Input: part model. Units: mm. Frame: model coordinates. A direction names the side the tool comes from. Give positions to 0.01 mm unless a question says otherwise; leave off trailing zeros. Loops run counter-clockwise (first coordinate to the right, second up) from the corner with the lowest first, then second, coordinate; pieces in that order, holes last. Notation, with made-up numbers: (87.25, 7) - (104.25, 7) arc R22 ccw to (104.25, 45) - close; hole circle Ø6 at (45.5, -37.5). An arc over 180 degrees is marked (long way). Answer as a JSON object with one key per item and string values.
from build123d import *

# Parameters (mm, degrees)
SKETCH1_7_W         = 63
SKETCH1_7_H         = 55
SKETCH1_7_R         = 1.5
SKETCH1_7_R_2       = 11.375
BOSS_EXTRUDE3_DEPTH = 10
BOSS_EXTRUDE4_START = -65
SKETCH1_8_W         = 63
SKETCH1_8_H         = 55
SKETCH1_8_R         = 1.5
SKETCH1_8_W_2       = 43
SKETCH1_8_H_2       = 43
BOSS_EXTRUDE4_DEPTH = 65
SKETCH4_W           = 12.5
SKETCH4_H           = 65
CUT_EXTRUDE5_DEPTH  = 6
SKETCH1_15_R        = 11.375
SKETCH1_15_R_2      = 4.375
BOSS_EXTRUDE5_DEPTH = 7
SKETCH1_16_R        = 11.375
SKETCH1_16_R_2      = 4.375
CUT_EXTRUDE7_DEPTH  = 3


with BuildPart() as part:
    # Sketch1<7> → Boss-Extrude3 (new body)
    with BuildSketch(Plane.XY):
        with Locations((21.5, 21.5)):
            Rectangle(SKETCH1_7_W, SKETCH1_7_H)
        with Locations((-5, 36.5)):
            Circle(SKETCH1_7_R, mode=Mode.SUBTRACT)
        with Locations((-5, 6.5)):
            Circle(SKETCH1_7_R, mode=Mode.SUBTRACT)
        with Locations((48, 6.5)):
            Circle(SKETCH1_7_R, mode=Mode.SUBTRACT)
        with Locations((48, 36.5)):
            Circle(SKETCH1_7_R, mode=Mode.SUBTRACT)
        with Locations((21.5, 21.5)):
            Circle(SKETCH1_7_R_2, mode=Mode.SUBTRACT)
    extrude(amount=BOSS_EXTRUDE3_DEPTH)

    # Sketch1<8> → Boss-Extrude4 (add)
    with BuildSketch(Plane.XY.offset(BOSS_EXTRUDE4_START)):
        with Locations((21.5, 21.5)):
            Rectangle(SKETCH1_8_W, SKETCH1_8_H)
        with Locations((48, 6.5)):
            Circle(SKETCH1_8_R, mode=Mode.SUBTRACT)
        with Locations((-5, 6.5)):
            Circle(SKETCH1_8_R, mode=Mode.SUBTRACT)
        with Locations((-5, 36.5)):
            Circle(SKETCH1_8_R, mode=Mode.SUBTRACT)
        with Locations((48, 36.5)):
            Circle(SKETCH1_8_R, mode=Mode.SUBTRACT)
        with Locations((21.5, 21.5)):
            Rectangle(SKETCH1_8_W_2, SKETCH1_8_H_2, mode=Mode.SUBTRACT)
    extrude(amount=BOSS_EXTRUDE4_DEPTH)

    # Sketch4 → Cut-Extrude5 (cut)
    with BuildSketch(Plane.XZ.offset(-43)):
        with Locations((27.75, -32.5)):
            Rectangle(SKETCH4_W, SKETCH4_H)
        with Locations((15.25, -32.5)):
            Rectangle(SKETCH4_W, SKETCH4_H)
    extrude(amount=-CUT_EXTRUDE5_DEPTH, mode=Mode.SUBTRACT)

    # Sketch1<15> → Boss-Extrude5 (add)
    with BuildSketch(Plane.XY):
        with Locations((21.5, 21.5)):
            Circle(SKETCH1_15_R)
        with Locations((21.5, 21.5)):
            Circle(SKETCH1_15_R_2, mode=Mode.SUBTRACT)
    extrude(amount=BOSS_EXTRUDE5_DEPTH)

    # Sketch1<16> → Cut-Extrude7 (cut)
    with BuildSketch(Plane.XY):
        with Locations((21.5, 21.5)):
            Circle(SKETCH1_16_R)
        with Locations((21.5, 21.5)):
            Circle(SKETCH1_16_R_2, mode=Mode.SUBTRACT)
    extrude(amount=CUT_EXTRUDE7_DEPTH, mode=Mode.SUBTRACT)


solid = part.part
Item 1: Cut plane D-D (y = 36.5). Return loops of the section in (x, z).
Geometry check:
{"outline": "(-10, -65) - (-6.5, -65) - (-6.5, 10) - (-10, 10) - close; (-3.5, -65) - (0, -65) - (0, 0) - (43, 0) - (43, -65) - (46.5, -65) - (46.5, 10) - (-3.5, 10) - close; (49.5, -65) - (53, -65) - (53, 10) - (49.5, 10) - close"}
Item 2: Material intervals for line 1 (Y direction, x = -5, z = -30); line 2 (X direction, y = 23.5, z = -30); line 3 (Y direction, x = 21.5, z = 1.8) (3 decimals), sorted ascending. Write a range as [from, to].
Geometry check:
{"line 1": "y = [-6, 5], [8, 35], [38, 49]", "line 2": "x = [-10, 0], [43, 53]", "line 3": "y = [-6, 10.125], [32.875, 49]"}
Item 3: Cut plane A-A (x = -5). Return loops of the section in (y, z).
Geometry check:
{"outline": "(-6, -65) - (5, -65) - (5, 10) - (-6, 10) - close; (8, -65) - (35, -65) - (35, 10) - (8, 10) - close; (38, -65) - (49, -65) - (49, 10) - (38, 10) - close"}
Item 4: Access query for faces 5 (the face through (9, 46, -33)), 6 (the face through (13.12, 29.19, 1.48)), 7 (the face through (-10, 21, -28)), 8 (the face through (26, 22, 7)). Directions: +Z, -Z, +X, -X, +Y, -Y. A direction counts if a zero-diameter tool reaches every point of the face in a straight line with its end or side. Return the directions, or none.
Geometry check:
{"face 5": "-Z, +Y", "face 6": "-Z", "face 7": "+Z, -Z, -X, +Y, -Y", "face 8": "+Z"}
Item 5: Mould query, pull axis Y, two halves, no side actions, for faces 1 (the face through (21, 34, 10)), 2 (the face through (26, 22, 3)), 3 (the face through (-5, 35, -28)), 4 (the face through (7, 49, -28)). Classes: released by +Y, released by -Y, zero draft, split by the parting line, or undercut.
Geometry check:
{"face 1": "zero draft", "face 2": "undercut", "face 3": "undercut", "face 4": "released by +Y"}
Item 6: Cut plane B-B (y = 21.5). Return loops of the section in (x, z) (3 decimals).
Geometry check:
{"outline": "(-10, -65) - (0, -65) - (0, 0) - (10.125, 0) - (10.125, 3) - (17.125, 3) - (17.125, 7) - (10.125, 7) - (10.125, 10) - (-10, 10) - close; (25.875, 3) - (32.875, 3) - (32.875, 0) - (43, 0) - (43, -65) - (53, -65) - (53, 10) - (32.875, 10) - (32.875, 7) - (25.875, 7) - close"}
Item 7: Contact query for flat-ended pins moving along their axis: P1, Ø11.5, axis at x = 26, y = 17, coming from the -Z side; P2, Ø13.5, axis at x = 21.5, y = 21.5, coming from the -Z side; P3, Ø4, axis at x = 27, z = -30, coming from the +Y side. Output: stop coordinate, or through.
Geometry check:
{"P1": "stops at z = 0", "P2": "stops at z = 3", "P3": "stops at y = 0"}
Item 8: Cut plane C-C (x = 21.5). Return loops of the section in (y, z) (3 decimals), then the cut area to 4 significant figures.
Geometry check:
{"outline": "(-6, -65) - (0, -65) - (0, 0) - (10.125, 0) - (10.125, 3) - (17.125, 3) - (17.125, 7) - (10.125, 7) - (10.125, 10) - (-6, 10) - close; (25.875, 3) - (32.875, 3) - (32.875, 0) - (49, 0) - (49, 10) - (32.875, 10) - (32.875, 7) - (25.875, 7) - close", "area": "768.5 mm2"}
